Design review of the part shown in the three views and the two pictorial views. Dimensions are in mm from the part's minimum x, y and z. A direction names the side the tool comes from. Give positions to 0.01 mm unless a question says otherwise; leave off trailing zeros. Loops run counter-clockwise (first coordinate to the right, second up) from the corner with the lowest first, then second, coordinate; pieces in that order, holes last. Notation, with made-up numbers: (83, -9) -> (120, -9) arc R17 cw to (120, 23) -> close; hole circle Ø9 at (4.25, 67). An arc over 180 degrees is marked (long way). Answer as CSV lines item,"result". Start each with the question number.
Item 1: For L1, parallel to X at y = 16.5, z = 4.25; L2, parallel to Y at x = 9, z = 7.5; L3, parallel to X at y = 20.5, z = 9, list the stretches that pass through material, from the lowest coordinate up. Write a range as from..to.
Item 2: Add section A-A on y = 16.38. State the section outline as (x, z) points (3 decimals), plus the area to 3 significant figures.
Item 3: Add section B-B on z = 4.5. State the section outline as (x, y) points (3 decimals), plus the area to 3 significant figures.
Item 4: The part is to be moulded in two halves that separate along Y. For the marked faces 4, 5 and 6, say which applies: +Y half, -Y half, draft (parallel to the pull), parting line (faces both ways), or undercut.
Item 5: Machinability: for the marked faces 1, 2 and 3, which of the approach directions +Z, -Z, +X, -X, +Y, -Y give a long, thin tool a straight path to every point of the face, cutting with its end or side? Answer none if there is none.
Item 6: Clearance check with flat-ended pins moving along their axes: P1, Ø2, axis at x = 34.5, y = 12, coming from the -Z side; P2, Ø3, axis at x = 42, z = 6.5, coming from the +Y side. State where each tip first meets the part, or that it passes through.
Item 7: Add section D-D on x = 27.5. State the section outline as (y, z) points, plus the area to 3 significant figures.
Item 8: Add section C-C on z = 9.25. State the section outline as (x, y) points (3 decimals).
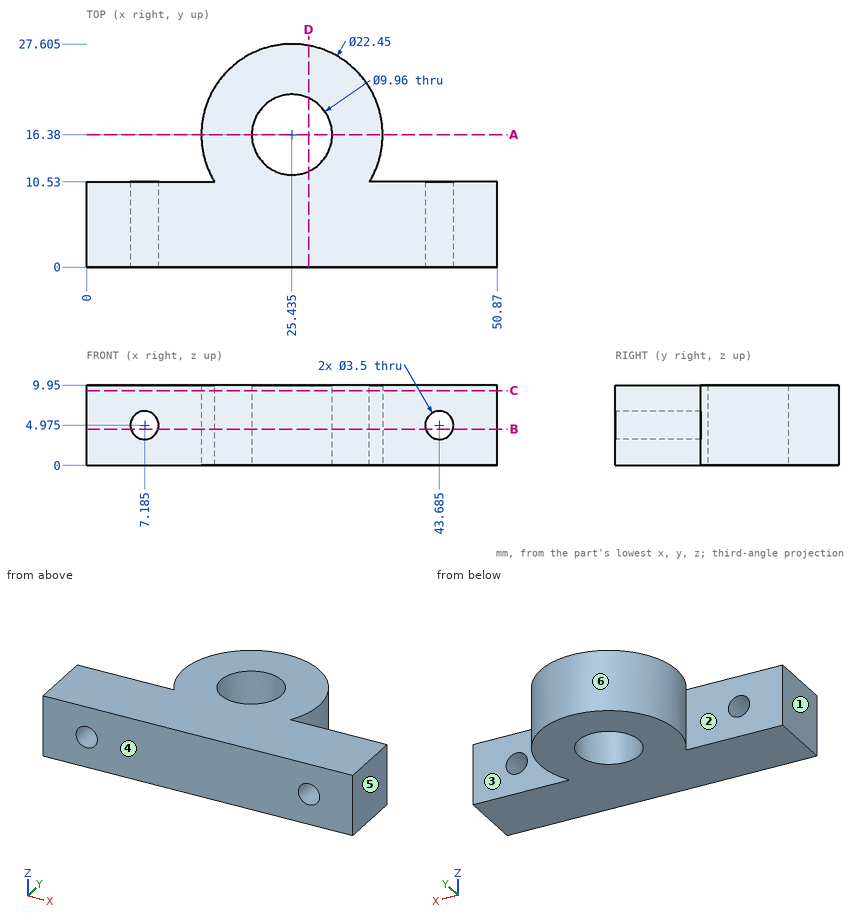
Computed values:
1,L1,"14.21..20.46, 30.41..36.66"
1,L2,"0..10.53"
1,L3,"14.99..22.64, 28.23..35.88"
2,outline,"(14.21, 0) -> (20.455, 0) -> (20.455, 9.95) -> (14.21, 9.95) -> close; (30.415, 0) -> (36.66, 0) -> (36.66, 9.95) -> (30.415, 9.95) -> close"
2,area,"124 mm²"
3,outline,"(0, 0) -> (5.501, 0) -> (5.501, 10.53) -> (0, 10.53) -> close; (8.869, 0) -> (42.001, 0) -> (42.001, 10.53) -> (35.015, 10.53) arc R11.225 ccw (long way) to (15.855, 10.53) -> (8.869, 10.53) -> close; (45.369, 0) -> (50.87, 0) -> (50.87, 10.53) -> (45.369, 10.53) -> close; hole circle Ø9.96 at (25.435, 16.38)"
3,area,"710 mm²"
4,face 4,"-Y half"
4,face 5,"draft"
4,face 6,"undercut"
5,face 1,"+Z, -Z, -X, +Y, -Y"
5,face 2,"+Z, -Z, -X"
5,face 3,"+Z, -Z, +X"
6,P1,"z = 0"
6,P2,"y = 10.53"
7,outline,"(0, 0) -> (11.85, 0) -> (11.85, 9.95) -> (0, 9.95) -> close; (20.91, 0) -> (27.41, 0) -> (27.41, 9.95) -> (20.91, 9.95) -> close"
7,area,"183 mm²"
8,outline,"(0, 0) -> (50.87, 0) -> (50.87, 10.53) -> (35.015, 10.53) arc R11.225 ccw (long way) to (15.855, 10.53) -> (0, 10.53) -> close; hole circle Ø9.96 at (25.435, 16.38)"
